Here's how the part is built. I have some questions about the finished solid (model axes, mm). A direction names the side the tool comes from. Round coordinates to 2 decimals unless told otherwise and drop trailing zeros. Write each loop counter-clockwise with the first axis right and the second up, starting at its lowest first coordinate (ties: lowest second). Pieces come first, ordered by that corner, then holes. Notation, with made-up numbers: (86.25, -35.5) - (115.25, -35.5) arc R27 ccw to (115.25, -16.5) - close; hole circle Ø8 at (54, 19.25). An arc over 180 degrees is marked (long way). One line per item, written item: value. Start each with the question number.
Item 1: Imagine slicing it at A-A, the plane x = -26.5. Please give me the cut outline in (y, z).
Item 2: Thinking about a two-plate mould opening in X: for faces 1 (the face through (-3, 0.5, -3)), 2 (the face through (-3, 0, -3)), 3 (the face through (-3, 150.5, -203)), 4 (the face through (221, 62, 3)), which applies, released by +X, released by -X, zero draft, split by the parting line, or undercut?
Item 3: Imagine slicing it at B-B, the plane z = -152. Please give me the cut outline in (x, y), then the cut area to 3 significant figures.
Item 4: If I drill on line 1 (X direction, y = 121.5, z = -132); line 2 (Y direction, x = 56.5, z = -46); line 3 (Z direction, x = 203, y = 22.5), over which ranges is the centre line in solid material (lowest first)?
Item 5: For P1, Ø10, axis at x = 117.5, y = 128, coming from the +Z side; P2, Ø9.5, axis at y = 160, z = -37, coming from the -X side; P3, Ø10, axis at x = -49, z = -69, coming from the +Y side, each with a flat end and sliding along its axis, tell me the tip position at first contact or that it passes through.
Item 6: For faces 5 (the face through (-3, 150, -202)), 6 (the face through (-218, 157, -7)), 7 (the face through (-221, 62, 3)), which set-ups out of +Z, -Z, +X, -X, +Y, -Y let a thin tool reach every point of the face, with its end or its side?
Item 7: Imagine slicing it at C-C, the plane y = 46.5. Please give me the cut outline in (x, z), then the cut area to 4 significant figures.
```python
from build123d import *

# Parameters (mm, degrees)
SKETCH1_W           = 442
SKETCH1_H           = 420
BOSS_EXTRUDE1_DEPTH = 0.5
SKETCH2_W           = 0.5
SKETCH2_H           = 420
BOSS_EXTRUDE2_DEPTH = 151
BOSS_EXTRUDE5_DEPTH = 408
BOSS_EXTRUDE3_DEPTH = 149.5
SKETCH41_W          = 3
SKETCH41_H          = 13
CUT_EXTRUDE1_DEPTH  = 3
SKETCH42_W          = 430
SKETCH42_H          = 0.5
BOSS_EXTRUDE6_DEPTH = 147.4
SKETCH43_W          = 429.998697479
SKETCH43_H          = 0.5
BOSS_EXTRUDE7_DEPTH = 15
SKETCH44_W          = 0.5
SKETCH44_H          = 12
BOSS_EXTRUDE8_DEPTH = 11.5
FILLET1_R           = 1
FILLET2_R           = 0.8


with BuildPart() as part:
    # Sketch1 → Boss-Extrude1 (new body)
    with BuildSketch(Plane(origin=(0, 0, 0), x_dir=(1, 0, 0), z_dir=(0, 1, 0))):
        Rectangle(SKETCH1_W, SKETCH1_H)
    extrude(amount=BOSS_EXTRUDE1_DEPTH)

    # Sketch2 → Boss-Extrude2 (add)
    with BuildSketch(Plane(origin=(0, 0.5, 0), x_dir=(1, 0, 0), z_dir=(0, 1, 0))):
        with Locations((-220.75, 0)):
            Rectangle(SKETCH2_W, SKETCH2_H)
        with Locations((220.75, 0)):
            Rectangle(SKETCH2_W, SKETCH2_H)
    extrude(amount=BOSS_EXTRUDE2_DEPTH)

    # Sketch39 → Boss-Extrude5 (add)
    with BuildSketch(Plane(origin=(0, 0, -210), x_dir=(-1, 0, 0), z_dir=(0, 0, -1))):
        Polygon((220.5, 151), (218, 151), (218, 163), (218.5, 163), (218.5, 151.5), (220.5, 151.5), align=None)
        Polygon((-220.5, 151.5), (-220.5, 151), (-218, 151), (-218, 163), (-218.5, 163), (-218.5, 151.5), align=None)
    extrude(amount=-BOSS_EXTRUDE5_DEPTH)

    # Sketch41 → Cut-Extrude1 (cut)
    with BuildSketch(Plane(origin=(0, 0, -210), x_dir=(-1, 0, 0), z_dir=(0, 0, -1))):
        with Locations((219.5, 156.5)):
            Rectangle(SKETCH41_W, SKETCH41_H)
        with Locations((-219.5, 156.5)):
            Rectangle(SKETCH41_W, SKETCH41_H)
    extrude(amount=-CUT_EXTRUDE1_DEPTH, mode=Mode.SUBTRACT)


with BuildPart() as body_2:
    # Sketch7 → Boss-Extrude3 (new body)
    with BuildSketch(Plane(origin=(0, 0.5, 0), x_dir=(1, 0, 0), z_dir=(0, 1, 0))):
        Polygon((-220.5, 210), (220.5, 210), (220.5, 199.5), (220, 199.5), (220, 209.5), (-220, 209.5), (-220, 199.5), (-220.5, 199.5), align=None)
    extrude(amount=BOSS_EXTRUDE3_DEPTH)


    add(part.part)  # Boss-Extrude6 merges part
    # Sketch42 → Boss-Extrude6 (add)
    with BuildSketch(Plane(origin=(0, 150, 0), x_dir=(1, 0, 0), z_dir=(0, 1, 0))):
        with Locations((0, 209.75)):
            Rectangle(SKETCH42_W, SKETCH42_H)
    extrude(amount=-BOSS_EXTRUDE6_DEPTH)

    # Sketch43 → Boss-Extrude7 (add)
    with BuildSketch(Plane.XY.offset(-210)):
        with Locations((-0.00065126, 150.25)):
            Rectangle(SKETCH43_W, SKETCH43_H)
    extrude(amount=BOSS_EXTRUDE7_DEPTH)

    # Sketch44 → Boss-Extrude8 (add)
    with BuildSketch(Plane(origin=(0, 151.5, 0), x_dir=(1, 0, 0), z_dir=(0, 1, 0))):
        with Locations((-220.75, -204)):
            Rectangle(SKETCH44_W, SKETCH44_H)
        with Locations((220.75, -204)):
            Rectangle(SKETCH44_W, SKETCH44_H)
    extrude(amount=BOSS_EXTRUDE8_DEPTH)

    # Fillet1
    fillet1_edges = [body_2.edges().sort_by_distance(p)[0] for p in [
        (-220.75, 163, 198),
        (220.75, 163, 198),
    ]]
    fillet(fillet1_edges, radius=FILLET1_R)

    # Fillet2
    fillet2_edges = [body_2.edges().sort_by_distance(p)[0] for p in [
        (-220.75, 151.5, 198),
        (220.75, 151.5, 198),
    ]]
    fillet(fillet2_edges, radius=FILLET2_R)


solid = body_2.part
```
Values follow:
1. outline: (0, -210) - (150.5, -210) - (150.5, -195) - (150, -195) - (150, -209.5) - (0.5, -209.5) - (0.5, 210) - (0, 210) - close
2. face 1: undercut
2. face 2: zero draft
2. face 3: undercut
2. face 4: released by +X
3. outline: (-221, 0) - (221, 0) - (221, 151.5) - (218.5, 151.5) - (218.5, 163) - (218, 163) - (218, 151) - (220.5, 151) - (220.5, 0.5) - (-220.5, 0.5) - (-220.5, 151) - (-218, 151) - (-218, 163) - (-218.5, 163) - (-218.5, 151.5) - (-221, 151.5) - close
3. area: 386 mm^2
4. line 1: x = -221 to -220.5, 220.5 to 221
4. line 2: y = 0 to 0.5
4. line 3: z = -210 to -209.5
5. P1: stops at z = -209.5
5. P2: stops at x = -218.5
5. P3: stops at y = 0.5
6. face 5: +Z
6. face 6: +Z, -Z, +Y
6. face 7: +Z, -Z, -X, +Y, -Y
7. outline: (-221, -210) - (221, -210) - (221, 210) - (220.5, 210) - (220.5, -199.5) - (220, -199.5) - (220, -209.5) - (-220, -209.5) - (-220, -199.5) - (-220.5, -199.5) - (-220.5, 210) - (-221, 210) - close
7. area: 650.5 mm^2
